```python
from build123d import *

# Parameters (mm, degrees)
F1_DEPTH = 6.35


with BuildPart() as f1:
    # F0 (on Front) → F1 (new body)
    with BuildSketch(Plane.XZ):
        with BuildLine():
            ThreePointArc((3.147837, 34.510579), (0, 31.75), (-3.147837, 34.510579))
            Line((-3.147837, 34.510579), (-4.022344, 36.290266))
            Line((-4.022344, 36.290266), (-5.520025, 36.093734))
            Line((-5.520025, 36.093734), (-5.891418, 34.14938))
            ThreePointArc((-5.891418, 34.14938), (-8.217505, 30.668145), (-11.972573, 32.51994))
            Line((-11.972573, 32.51994), (-13.277898, 34.012646))
            Line((-13.277898, 34.012646), (-14.673681, 33.435182))
            Line((-14.673681, 33.435182), (-14.529182, 31.460957))
            ThreePointArc((-14.529182, 31.460957), (-15.875, 27.496307), (-19.981397, 28.31312))
            Line((-19.981397, 28.31312), (-21.628585, 29.41712))
            Line((-21.628585, 29.41712), (-22.827349, 28.498078))
            Line((-22.827349, 28.498078), (-22.176807, 26.628522))
            ThreePointArc((-22.176807, 26.628522), (-22.45064, 22.45064), (-26.628522, 22.176807))
            Line((-26.628522, 22.176807), (-28.50532, 22.816867))
            Line((-28.50532, 22.816867), (-29.425371, 21.618877))
            Line((-29.425371, 21.618877), (-28.31312, 19.981397))
            ThreePointArc((-28.31312, 19.981397), (-27.496307, 15.875), (-31.460957, 14.529182))
            Line((-31.460957, 14.529182), (-33.439464, 14.661681))
            Line((-33.439464, 14.661681), (-34.018103, 13.266385))
            Line((-34.018103, 13.266385), (-32.51994, 11.972573))
            ThreePointArc((-32.51994, 11.972573), (-30.668145, 8.217505), (-34.14938, 5.891418))
            Line((-34.14938, 5.891418), (-36.094764, 5.507326))
            Line((-36.094764, 5.507326), (-36.292557, 4.009811))
            Line((-36.292557, 4.009811), (-34.510579, 3.147837))
            ThreePointArc((-34.510579, 3.147837), (-31.75, 0), (-34.510579, -3.147837))
            Line((-34.510579, -3.147837), (-36.290266, -4.022344))
            Line((-36.290266, -4.022344), (-36.093734, -5.520025))
            Line((-36.093734, -5.520025), (-34.14938, -5.891418))
            ThreePointArc((-34.14938, -5.891418), (-30.668145, -8.217505), (-32.51994, -11.972573))
            Line((-32.51994, -11.972573), (-34.012646, -13.277898))
            Line((-34.012646, -13.277898), (-33.435182, -14.673681))
            Line((-33.435182, -14.673681), (-31.460957, -14.529182))
            ThreePointArc((-31.460957, -14.529182), (-27.496307, -15.875), (-28.31312, -19.981397))
            Line((-28.31312, -19.981397), (-29.41712, -21.628585))
            Line((-29.41712, -21.628585), (-28.498078, -22.827349))
            Line((-28.498078, -22.827349), (-26.628522, -22.176807))
            ThreePointArc((-26.628522, -22.176807), (-22.45064, -22.45064), (-22.176807, -26.628522))
            Line((-22.176807, -26.628522), (-22.816867, -28.50532))
            Line((-22.816867, -28.50532), (-21.618877, -29.425371))
            Line((-21.618877, -29.425371), (-19.981397, -28.31312))
            ThreePointArc((-19.981397, -28.31312), (-15.875, -27.496307), (-14.529182, -31.460957))
            Line((-14.529182, -31.460957), (-14.661681, -33.439464))
            Line((-14.661681, -33.439464), (-13.266385, -34.018103))
            Line((-13.266385, -34.018103), (-11.972573, -32.51994))
            ThreePointArc((-11.972573, -32.51994), (-8.217505, -30.668145), (-5.891418, -34.14938))
            Line((-5.891418, -34.14938), (-5.507326, -36.094764))
            Line((-5.507326, -36.094764), (-4.009811, -36.292557))
            Line((-4.009811, -36.292557), (-3.147837, -34.510579))
            ThreePointArc((-3.147837, -34.510579), (0, -31.75), (3.147837, -34.510579))
            Line((3.147837, -34.510579), (4.022344, -36.290266))
            Line((4.022344, -36.290266), (5.520025, -36.093734))
            Line((5.520025, -36.093734), (5.891418, -34.14938))
            ThreePointArc((5.891418, -34.14938), (8.217505, -30.668145), (11.972573, -32.51994))
            Line((11.972573, -32.51994), (13.277898, -34.012646))
            Line((13.277898, -34.012646), (14.673681, -33.435182))
            Line((14.673681, -33.435182), (14.529182, -31.460957))
            ThreePointArc((14.529182, -31.460957), (15.875, -27.496307), (19.981397, -28.31312))
            Line((19.981397, -28.31312), (21.628585, -29.41712))
            Line((21.628585, -29.41712), (22.827349, -28.498078))
            Line((22.827349, -28.498078), (22.176807, -26.628522))
            ThreePointArc((22.176807, -26.628522), (22.45064, -22.45064), (26.628522, -22.176807))
            Line((26.628522, -22.176807), (28.50532, -22.816867))
            Line((28.50532, -22.816867), (29.425371, -21.618877))
            Line((29.425371, -21.618877), (28.31312, -19.981397))
            ThreePointArc((28.31312, -19.981397), (27.496307, -15.875), (31.460957, -14.529182))
            Line((31.460957, -14.529182), (33.439464, -14.661681))
            Line((33.439464, -14.661681), (34.018103, -13.266385))
            Line((34.018103, -13.266385), (32.51994, -11.972573))
            ThreePointArc((32.51994, -11.972573), (30.668145, -8.217505), (34.14938, -5.891418))
            Line((34.14938, -5.891418), (36.094764, -5.507326))
            Line((36.094764, -5.507326), (36.292557, -4.009811))
            Line((36.292557, -4.009811), (34.510579, -3.147837))
            ThreePointArc((34.510579, -3.147837), (31.75, 0), (34.510579, 3.147837))
            Line((34.510579, 3.147837), (36.290266, 4.022344))
            Line((36.290266, 4.022344), (36.093734, 5.520025))
            Line((36.093734, 5.520025), (34.14938, 5.891418))
            ThreePointArc((34.14938, 5.891418), (30.668145, 8.217505), (32.51994, 11.972573))
            Line((32.51994, 11.972573), (34.012646, 13.277898))
            Line((34.012646, 13.277898), (33.435182, 14.673681))
            Line((33.435182, 14.673681), (31.460957, 14.529182))
            ThreePointArc((31.460957, 14.529182), (27.496307, 15.875), (28.31312, 19.981397))
            Line((28.31312, 19.981397), (29.41712, 21.628585))
            Line((29.41712, 21.628585), (28.498078, 22.827349))
            Line((28.498078, 22.827349), (26.628522, 22.176807))
            ThreePointArc((26.628522, 22.176807), (22.45064, 22.45064), (22.176807, 26.628522))
            Line((22.176807, 26.628522), (22.816867, 28.50532))
            Line((22.816867, 28.50532), (21.618877, 29.425371))
            Line((21.618877, 29.425371), (19.981397, 28.31312))
            ThreePointArc((19.981397, 28.31312), (15.875, 27.496307), (14.529182, 31.460957))
            Line((14.529182, 31.460957), (14.661681, 33.439464))
            Line((14.661681, 33.439464), (13.266385, 34.018103))
            Line((13.266385, 34.018103), (11.972573, 32.51994))
            ThreePointArc((11.972573, 32.51994), (8.217505, 30.668145), (5.891418, 34.14938))
            Line((5.891418, 34.14938), (5.507326, 36.094764))
            Line((5.507326, 36.094764), (4.009811, 36.292557))
            Line((4.009811, 36.292557), (3.147837, 34.510579))
        make_face()
        with BuildLine():
            ThreePointArc((1.524, 6.164408), (0.065583, -6.349661), (-1.651, 6.131615))
            Line((-1.651, 6.131615), (-1.651, 7.739208))
            Line((-1.651, 7.739208), (1.524, 7.739208))
            Line((1.524, 7.739208), (1.524, 6.164408))
        make_face(mode=Mode.SUBTRACT)
    extrude(amount=F1_DEPTH)


solid = f1.part
```
Geometry check sheet. Reference: the model listing, model coordinates, mm. A direction names the side the tool comes from. Round coordinates to 2 decimals unless told otherwise and drop trailing zeros. Loops run counter-clockwise (first coordinate to the right, second up) from the corner with the lowest first, then second, coordinate; pieces in that order, holes last. Notation, with made-up numbers: (-25.5, -39) -> (-15.5, -39) arc R37 cw to (-15.5, -2) -> close; hole circle Ø9 at (31, 6). An arc over 180 degrees is marked (long way). Use a Markdown table: item, result.
(1) Sectioned sample at C-C (x = 18.5). Enter the section's corners in (y, z), then the cut area to 3 significant figures.
Calculated:
| item | result |
|---|---|
| outline | (-6.35, -27.25) -> (0, -27.25) -> (0, 27.25) -> (-6.35, 27.25) -> close |
| area | 346 mm² |
(2) Sectioned sample at B-B (z = 0). Enter the section's corners in (x, y).
Calculated:
| item | result |
|---|---|
| outline | (-31.75, -6.35) -> (-6.35, -6.35) -> (-6.35, 0) -> (-31.75, 0) -> close; (6.35, -6.35) -> (31.75, -6.35) -> (31.75, 0) -> (6.35, 0) -> close |
(3) Scan lines: probe 1 along Z at (x, y) = (-32, -3.25); probe 2 along X at (y, z) = (-2, -17.5); probe 3 along X at (y, z) = (-3, 20). Record each from-to range of solid material in increasing order.
Calculated:
| item | result |
|---|---|
| probe 1 | -14.57 to -11.7, -6.38 to -1.23, 1.23 to 6.38, 11.7 to 14.57 |
| probe 2 | -27.07 to 27.07 |
| probe 3 | -28.33 to 28.33 |
(4) Mould release check, pull along Z, two halves, no side actions. Record for faces 4 (the cylindrical face through (-30.685, -3.131, -8.156)), 5 (the flat face through (28.857, -3.131, 20.793)), 6 (the flat face through (20.812, -3.131, 28.877)), 7 (the flat face through (-32.462, -3.131, -14.602)): released by +Z, released by -Z, zero draft, split by the parting line, or undercut.
Calculated:
| item | result |
|---|---|
| face 4 | undercut |
| face 5 | undercut |
| face 6 | released by +Z |
| face 7 | released by -Z |
(5) Sectioned sample at D-D (z = 24.5). Enter the section's corners in (x, y).
Calculated:
| item | result |
|---|---|
| outline | (-21.53, -6.35) -> (21.53, -6.35) -> (21.53, 0) -> (-21.53, 0) -> close |
(6) Sectioned sample at A-A (x = 0). Enter the section's corners in (y, z).
Calculated:
| item | result |
|---|---|
| outline | (-6.35, -31.75) -> (0, -31.75) -> (0, -6.35) -> (-6.35, -6.35) -> close; (-6.35, 7.74) -> (0, 7.74) -> (0, 31.75) -> (-6.35, 31.75) -> close |
(7) Set-up check for faces 1 (the flat face through (3.585, -3.131, 35.414)), 2 (the flat face through (-3.585, -3.131, -35.414)), 3 (the flat face through (-14.595, -3.131, -32.436)): record each of +Z, -Z, +X, -X, +Y, -Y from which the full face is reachable in a straight line by a thin tool's end or side.
Calculated:
| item | result |
|---|---|
| face 1 | +Z, +Y, -Y |
| face 2 | -Z, +Y, -Y |
| face 3 | -X, +Y, -Y |
(8) Go/stop test with flat-tipped pins: P1, Ø0.5, axis at y = -2.5, z = 6.5, coming from the +X side; P2, Ø1.5, axis at y = -3.5, z = 16, coming from the -X side; P3, Ø1, axis at x = -24.5, y = -0.5, coming from the -Z side. Record where each tip stops, or that it passes through.
Calculated:
| item | result |
|---|---|
| P1 | x = 32.22 |
| P2 | x = -27.97 |
| P3 | z = -21.6 |
